Read the model definition and answer for the solid it produces. Units are mm, in the model's axes. A direction names the side the tool comes from. Coordinates: 2 decimals unless noted, no trailing zeros. Write each loop counter-clockwise with the first axis right and the second up, starting at its lowest first coordinate (ties: lowest second). Pieces come first, ordered by that corner, then holes. Notation, with made-up numbers: (67, -10.75) -> (126, -10.75) arc R21 cw to (126, -1.75) -> close; hole circle Ø1 at (-21.5, 64). An arc over 180 degrees is marked (long way). Answer in a Markdown table with one row per item. Add a question column.
Item 1: Straight lines are drawn through the part: line 1 (Y direction, x = 0.65, z = -26.1); line 2 (Z direction, x = 1.75, y = 4); line 3 (X direction, y = 17, z = 13). For each, find the intervals that lie inside material, in ascending order. Write a range as from..to.
Item 2: Which of the six approach directions +Z, -Z, +X, -X, +Y, -Y give full straight-line access (tool end or side, diameter ignored) to faces 1 (the face through (1, 30.5, -33)), 2 (the face through (5, 30.5, 24)), 3 (the face through (6, 2, 18.8)), 4 (the face through (3, 2, 27.1)), 5 (the face through (1, 4.5, -33))?
Item 3: Section D-D on y = 11 is taken. Write down the section's boundary in (x, z).
Item 4: Section B-B on z = 26.1 is taken. Write down the section's boundary in (x, y).
Item 5: Given pin 1 Ø0.8 at (x, z) = (1.5, 31.5) entering from +Y; pin 2 Ø3.5 at (y, z) = (32, 20.5) entering from -X; pin 3 Ø1.4 at (x, y) = (3, 33.5) entering from +Z; pin 4 Ø2.5 at (y, z) = (17.5, 26.1) entering from -X, each flat-ended and moving along its own axis, determine where each tip first touches the part or whether it passes through.
Item 6: Section A-A on y = 17.5 is taken. Write down the section's boundary in (x, z), then the cut area to 4 significant figures.
Item 7: For a pull along X with two mould halves and no side action, classify faces 6 (the face through (6.8, 33, -23)), 7 (the face through (3, 33, 24.6)), 8 (the face through (5, 4.5, -24)), 9 (the face through (3, 2, -24.6)) as +X half, -X half, draft (parallel to the pull), parting line (faces both ways), or undercut.
Autodesk Inventor part; units mm, degrees
ref_plane "YZ Plane" through (0, 0, 0) normal (1, 0, 0) x (0, 1, 0)
ref_plane "XZ Plane" through (0, 0, 0) normal (0, 1, 0) x (-1, 0, 0)
ref_plane "XY Plane" through (0, 0, 0) normal (0, 0, 1) x (1, 0, 0)
sketch "Sketch1" plane through (0, 0, 0) normal (0, 1, 0) x (-1, 0, 0)
  line L0 (0, 27.1) -> (0, -27.1)
  line L1 (0, 27.1) -> (-6.8, 27.1)
  line L2 (-6.8, 27.1) -> (-6.8, 18.8)
  line L3 (-6.8, 18.8) -> (-4.3, 18.8)
  line L4 (-4.3, 18.8) -> (-4.3, 24.6)
  line L5 (-4.3, 24.6) -> (-2.5, 24.6)
  line L6 (-2.5, 24.6) -> (-2.5, 0)
  line L7 (0, -27.1) -> (-6.8, -27.1)
  line L8 (-6.8, -27.1) -> (-6.8, -18.8)
  line L9 (-6.8, -18.8) -> (-4.3, -18.8)
  line L10 (-4.3, -18.8) -> (-4.3, -24.6)
  line L11 (-4.3, -24.6) -> (-2.5, -24.6)
  line L12 (-2.5, -24.6) -> (-2.5, 0)
  point P0 (0, 0)
  dimension "d0" = 54.2
  dimension "d1" = 6.8
  dimension "d2" = 8.3
  dimension "d3" = 2.5
  dimension "d4" = 5.8
  dimension "d5" = 1.8
  dimension "d6" = 8.3
  dimension "d7" = 5.8
extrude "Extrusion1" add sketch "Sketch1" along normal blind 4.5
sketch "Sketch2" plane through (0, 4.5, 0) normal (0, 1, 0) x (1, 0, 0)
  line L0 (2.5, -24.6) -> (2.5, 24.6)
  line L1 (2.5, 0) -> (2.5, 39.5)
  line L2 (2.5, 39.5) -> (0, 39.5)
  line L3 (0, 39.5) -> (0, 0)
  line L4 (0, 0) -> (0, -39.5)
  line L5 (0, 27.1) -> (0, -27.1)
  line L6 (0, -39.5) -> (2.5, -39.5)
  line L7 (2.5, -39.5) -> (2.5, 0)
  dimension "d10" = 39.5
  dimension "d11" = 39.5
extrude "Extrusion2" add sketch "Sketch2" along normal blind 26
sketch "Sketch3" plane through (0, 30.5, 0) normal (0, 1, 0) x (1, 0, 0)
  line L0 (2.5, -24.6) -> (2.5, 24.6)
  line L1 (2.5, 0) -> (2.5, 24.6558)
  line L2 (0, 27.1) -> (0, -27.1)
  line L3 (4.3, -24.6) -> (2.5, -24.6)
  line L4 (6.8, -18.8) -> (4.3, -18.8)
  line L5 (4.3, -24.6) -> (4.3, -18.8)
  line L6 (4.3, -18.8) -> (6.8, -18.8)
  line L7 (6.8, -18.8) -> (6.8, -27.1)
  line L8 (6.8, -27.1) -> (2.5, -27.1)
  line L9 (2.5, 0) -> (2.5, 24.6558)
  line L10 (2.5, 24.6) -> (4.3, 24.6)
  line L11 (4.3, 18.8) -> (6.8, 18.8)
  line L12 (4.3, 24.6) -> (4.3, 18.8)
  line L13 (4.3, 18.8) -> (6.8, 18.8)
  line L14 (6.8, 18.8) -> (6.8, 27.1)
  line L15 (6.8, 27.1) -> (0, 27.1)
  line L16 (0, 27.1) -> (0, -27.1)
  line L17 (6.8, -27.1) -> (0, -27.1)
  line L18 (4.3, -24.6) -> (2.5, -24.6)
  point P0 (0, 0)
extrude "Extrusion3" add sketch "Sketch3" along normal blind 4.5
sketch "Sketch4" plane through (2.5, 0, 24.6) normal (1, 0, 0) x (0, 0, -1)
  line L0 (64.1, 4.5) -> (64.1, 30.5)
  line L1 (64.1, 17.5) -> (50.7, 17.5)
  circle A0 centre (50.7, 17.5) radius 1.5
  line L2 (-14.9, 4.5) -> (-14.9, 30.5)
  line L3 (-14.9, 17.5) -> (-1.5, 17.5)
  circle A1 centre (-1.5, 17.5) radius 1.5
  point P0 (24.6, 0)
  dimension "d16" = 13.4
  dimension "d17" = 3
  dimension "d18" = 13.4
  dimension "d19" = 3
extrude "Extrusion4" cut sketch "Sketch4" against normal blind 4.5
properties part number "cam_holder2_conv"
Results below:
| question | item | result |
|---|---|---|
| 1 | line 1 | y = 0..16, 19..35 |
| 1 | line 2 | z = -27.1..27.1 |
| 1 | line 3 | x = 0..2.5 |
| 2 | face 1 | -Z, +X, -X, +Y |
| 2 | face 2 | +Z, -Z, +X |
| 2 | face 3 | +X, +Y, -Y |
| 2 | face 4 | +Z, +X, -X, -Y |
| 2 | face 5 | -Z, +X, -X, -Y |
| 3 | outline | (0, -39.5) -> (2.5, -39.5) -> (2.5, 39.5) -> (0, 39.5) -> close |
| 4 | outline | (0, 0) -> (6.8, 0) -> (6.8, 4.5) -> (2.5, 4.5) -> (2.5, 16) -> (0, 16) -> close; (0, 19) -> (2.5, 19) -> (2.5, 30.5) -> (6.8, 30.5) -> (6.8, 35) -> (0, 35) -> close |
| 5 | pin 1 | stops at y = 30.5 |
| 5 | pin 2 | stops at x = 0 |
| 5 | pin 3 | stops at z = 27.1 |
| 5 | pin 4 | passes through |
| 6 | outline | (0, -39.5) -> (2.5, -39.5) -> (2.5, -27.6) -> (0, -27.6) -> close; (0, -24.6) -> (2.5, -24.6) -> (2.5, 24.6) -> (0, 24.6) -> close; (0, 27.6) -> (2.5, 27.6) -> (2.5, 39.5) -> (0, 39.5) -> close |
| 6 | area | 182.5 mm2 |
| 7 | face 6 | +X half |
| 7 | face 7 | undercut |
| 7 | face 8 | draft |
| 7 | face 9 | undercut |
